For this review, take the finished solid that the model builds, in its own axes (mm). A direction names the side the tool comes from. Round coordinates to 2 decimals unless told otherwise and drop trailing zeros. Write each loop counter-clockwise with the first axis right and the second up, starting at its lowest first coordinate (ties: lowest second). Pieces come first, ordered by that corner, then holes. Notation, with made-up numbers: (34.25, 25) - (87.25, 25) arc R21 cw to (87.25, 36) - close; hole circle Ø9 at (-33, 81.25). An arc over 180 degrees is marked (long way). One line per item, written item: value. Start each with the question number.
Q1. Add section C-C on z = 92. Write out the cut boundary in (x, y).
Q2. Add section D-D on y = -63.5. Write out the cut boundary in (x, z), and give its area (3 significant figures).
Q3. Clearance check with flat-ended pins moving along their axes: pin 1 Ø8 at (x, z) = (-65.5, 173.5) entering from +Y; pin 2 Ø12 at (x, y) = (-36, 50.5) entering from -Z; pin 3 Ø5 at (y, z) = (2.5, 83) entering from -X. State where each tip first meets the part, or that it passes through.
Q4. Add section B-B on y = 0. Write out the cut boundary in (x, z), and give its area (4 significant figures).
Q5. Tool access review of faces 4 (the face through (47.69, 15.02, 176.05)), 5 (the face through (1.75, 22.528, -71.537)), 6 (the face through (-125, 1, 1)): name each direction out of +Z, -Z, +X, -X, +Y, -Y from which nothing blocks a thin tool from reaching the whole face with its end or side.
Q6. Add section A-A on x = 0. Write out the cut boundary in (y, z).
Q7. Mouldability with a two-part tool opening along X and no side actions: class faces 1 (the face through (49, 16, 250)), 2 (the face through (-1, 1, 100)), 3 (the face through (125, 1, 1)) as +X half, -X half, draft (parallel to the pull), parting line (faces both ways), or undercut.
Q8. For probe 1 along Y at (x, z) = (24, 198); probe 2 along Y at (x, z) = (-32, 165.5); probe 3 along Z at (x, y) = (-72, -3), list the stretches that pass through material, from the lowest coordinate up.
```python
from build123d import *

# Parameters (mm, degrees)
SKETCH1_R           = 75
BOSS_EXTRUDE1_DEPTH = 125
SKETCH2_R           = 75
BOSS_EXTRUDE2_DEPTH = 250
SKETCH3_R           = 50
CUT_EXTRUDE1_DEPTH  = 150


with BuildPart() as part:
    # Sketch1 → Boss-Extrude1 (new, symmetric)
    with BuildSketch(Plane(origin=(0, 0, 0), x_dir=(0, 0, -1), z_dir=(1, 0, 0))):
        Circle(SKETCH1_R)
    extrude(amount=BOSS_EXTRUDE1_DEPTH, both=True)

    # Sketch2 → Boss-Extrude2 (add)
    with BuildSketch(Plane.XY):
        with Locations(Location((0, 0, 0), (0, 0, 90))):
            Circle(SKETCH2_R)
    extrude(amount=BOSS_EXTRUDE2_DEPTH)

    # Sketch3 → Cut-Extrude1 (cut)
    with BuildSketch(Plane.XY.offset(250)):
        Circle(SKETCH3_R)
    extrude(amount=-CUT_EXTRUDE1_DEPTH, mode=Mode.SUBTRACT)


solid = part.part
```
Result set:
1. outline: circle Ø150 at (0, 0)
2. outline: (-125, -39.91) - (125, -39.91) - (125, 39.91) - (39.91, 39.91) - (39.91, 250) - (-39.91, 250) - (-39.91, 39.91) - (-125, 39.91) - close
2. area: 36,700 mm^2
3. pin 1: stops at y = 42.93
3. pin 2: stops at z = -60.37
3. pin 3: stops at x = -75
4. outline: (-125, -75) - (125, -75) - (125, 75) - (75, 75) - (75, 250) - (50, 250) - (50, 100) - (-50, 100) - (-50, 250) - (-75, 250) - (-75, 75) - (-125, 75) - close
4. area: 48,750 mm^2
5. face 4: +Z
5. face 5: none
5. face 6: +Z, -Z, -X, +Y, -Y
6. outline: (-75, 0) arc R75 ccw to (75, 0) - (75, 250) - (50, 250) - (50, 100) - (-50, 100) - (-50, 250) - (-75, 250) - close
7. face 1: draft
7. face 2: undercut
7. face 3: +X half
8. probe 1: y = -71.06 to -43.86, 43.86 to 71.06
8. probe 2: y = -67.83 to -38.42, 38.42 to 67.83
8. probe 3: z = -74.94 to 250
